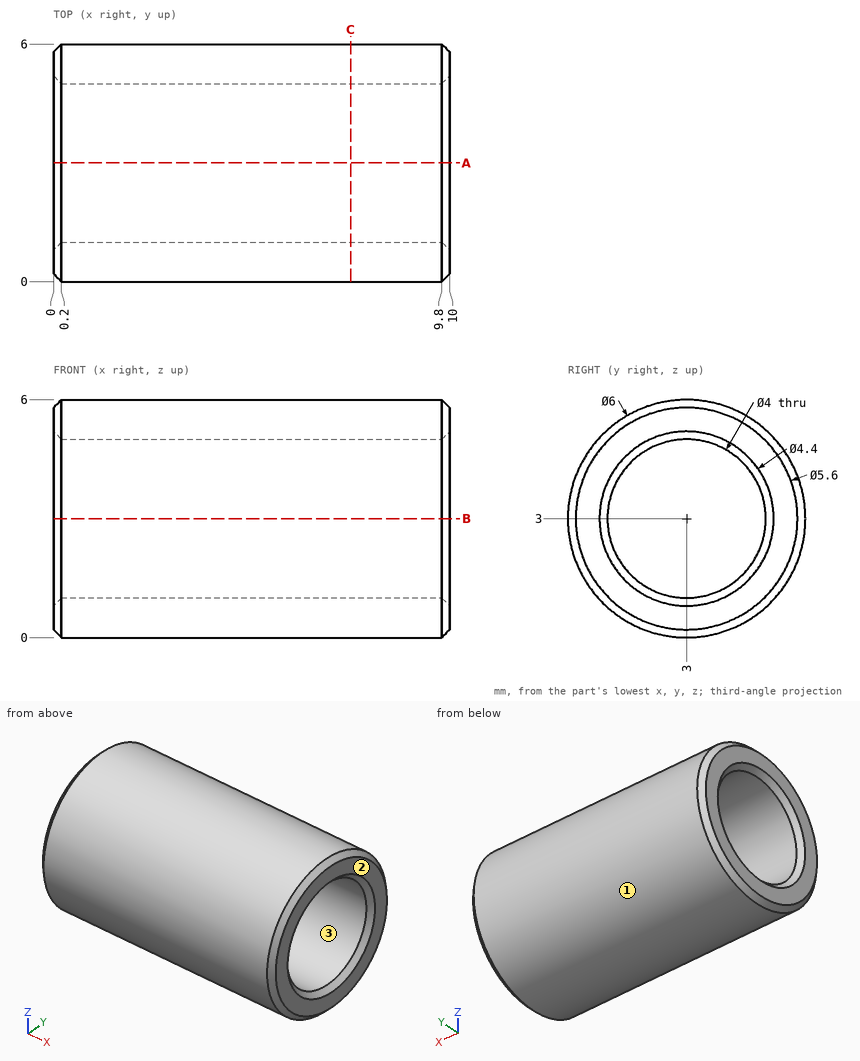
Could you check a few things on this drawing? It's one solid part, dimensions in mm from its lowest x, y, z. Give positions to 0.01 mm unless a question says otherwise; leave off trailing zeros. Write each loop counter-clockwise with the first axis right and the second up, starting at its lowest first coordinate (ties: lowest second). Pieces come first, ordered by that corner, then holes. Notation, with made-up numbers: (40.5, 27.5) -> (76.5, 27.5) arc R18 cw to (76.5, 39.5) -> close; hole circle Ø7 at (-5, 54.5). An arc over 180 degrees is marked (long way). Answer as CSV lines item,"result". Start each with the question number.
(1) Please list where these lines run through material, in increasing order: line 1 (Y direction, x = 9.25, z = 2.9); line 2 (Y direction, x = 1.5, z = 1.7).
(2) If we section it at C-C, the plane x = 7.5: Write out the boundary of the cut face in (y, z).
(3) If we mould it in two halves opening along Y, with no side actions, what happens to the marked faces 1, 2 and 3? For each: +Y half, -Y half, draft (parallel to the pull), parting line (faces both ways), or undercut.
(4) If we section it at A-A, the plane y = 3: Write out the boundary of the cut face in (x, z), and give its area (3 significant figures).
(5) I'm going to push flat-ended pins straight in: pin 1 Ø1 at (x, y) = (3, 4) entering from -Z; pin 2 Ø2 at (x, z) = (3, 4) entering from +Y. Where does each tip first touch, or does it pass through?
Answer list:
1,line 1,"0 to 1, 5 to 6"
1,line 2,"0.3 to 1.48, 4.52 to 5.7"
2,outline,"circle Ø6 at (3, 3); hole circle Ø4 at (3, 3)"
3,face 1,"parting line"
3,face 2,"draft"
3,face 3,"undercut"
4,outline,"(0, 0.2) -> (0.2, 0) -> (9.8, 0) -> (10, 0.2) -> (10, 0.8) -> (9.8, 1) -> (0.2, 1) -> (0, 0.8) -> close; (0, 5.2) -> (0.2, 5) -> (9.8, 5) -> (10, 5.2) -> (10, 5.8) -> (9.8, 6) -> (0.2, 6) -> (0, 5.8) -> close"
4,area,"19.8 mm^2"
5,pin 1,"z = 0.04"
5,pin 2,"y = 6"
